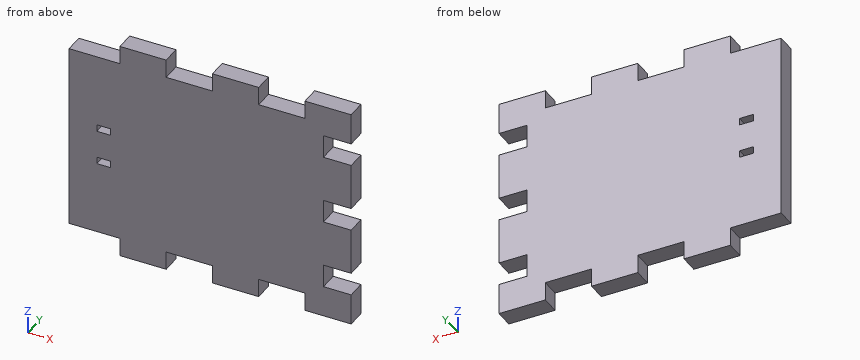
```python
from build123d import *

# Parameters (mm, degrees)
SKETCH1_W           = 55
SKETCH1_H           = 40.5
BOSS_EXTRUDE1_DEPTH = 4
SKETCH2_W           = 2.75
SKETCH2_H           = 4
SKETCH2_W_2         = 10
BOSS_EXTRUDE2_DEPTH = 6
SKETCH3_W           = 10
SKETCH3_H           = 4
BOSS_EXTRUDE3_DEPTH = 4
LPATTERN1_COUNT     = 3
LPATTERN1_PITCH     = 20
SKETCH4_W           = 3
SKETCH4_H           = 1.5
CUT_EXTRUDE1_DEPTH  = 5


with BuildPart() as part:
    # Sketch1 → Boss-Extrude1 (new body)
    with BuildSketch(Plane(origin=(0, 0, 0), x_dir=(1, 0, 0), z_dir=(0, 1, 0))):
        with Locations((27.5, -20.25)):
            Rectangle(SKETCH1_W, SKETCH1_H)
    extrude(amount=BOSS_EXTRUDE1_DEPTH)

    # Sketch2 → Boss-Extrude2 (add)
    with BuildSketch(Plane(origin=(55, 0, 0), x_dir=(0, 0, -1), z_dir=(1, 0, 0))):
        with Locations((-39.125, 2)):
            Rectangle(SKETCH2_W, SKETCH2_H)
        with Locations((-27.75, 2)):
            Rectangle(SKETCH2_W_2, SKETCH2_H)
        with Locations((-12.75, 2)):
            Rectangle(SKETCH2_W_2, SKETCH2_H)
        with Locations((-1.375, 2)):
            Rectangle(SKETCH2_W, SKETCH2_H)
    extrude(amount=BOSS_EXTRUDE2_DEPTH)

    # Sketch3 → Boss-Extrude3 (add, through all)
    with BuildSketch(Plane(origin=(0, 4, 0), x_dir=(1, 0, 0), z_dir=(0, 1, 0))):
        with Locations((56, 2)):
            Rectangle(SKETCH3_W, SKETCH3_H)
        with Locations((56, -42.5)):
            Rectangle(SKETCH3_W, SKETCH3_H)
    boss_extrude3 = extrude(amount=-BOSS_EXTRUDE3_DEPTH)

    # LPattern1: Boss-Extrude3 ×3
    with Locations(*[(-i * LPATTERN1_PITCH, 0, 0) for i in range(1, LPATTERN1_COUNT)]):
        add(boss_extrude3)

    # Sketch4 → Cut-Extrude1 (cut, through all)
    with BuildSketch(Plane(origin=(0, 4, 0), x_dir=(1, 0, 0), z_dir=(0, 1, 0))):
        with Locations((7.5, -24)):
            Rectangle(SKETCH4_W, SKETCH4_H)
        with Locations((7.5, -16.5)):
            Rectangle(SKETCH4_W, SKETCH4_H)
    extrude(amount=-CUT_EXTRUDE1_DEPTH, mode=Mode.SUBTRACT)


solid = part.part
```
Geometry check sheet. Reference: the model listing, model coordinates, mm. Round coordinates to 2 decimals unless told otherwise and drop trailing zeros. Order: outer loops, then holes, each group sorted by start corner. A loop starts at its lowest first (then second) coordinate and runs counter-clockwise, first axis right, second up. Notation, with made-up numbers: (55, 29) - (66, 29) arc R22 ccw to (66, 51) - close; hole circle Ø2 at (0.25, 4). An arc over 180 degrees is marked (long way). Use a Markdown table: item, result. Add a question column.
1) Section check B-B (x = 22.5). Record the cut outline in (y, z), then the cut area to 3 significant figures.
2) Thickness scan on line 1 along X through (y, z) = (3.4, 42.5); line 2 along Z through (x, y) = (7, 0.85); line 3 along X through (y, z) = (2.7, 17). Record the ranges inside material, lowest first.
3) Section check A-A (y = 1.2). Count the separate pieces of the cut face and the enclosed holes in it, then the cut area to 3 significant figures.
4) Section check C-C (z = 35). Record the cut outline in (x, y), then the cut area to 3 significant figures.
5) Gauge pin test, flat ends, axial feed: P1, Ø8, axis at x = 26.5, z = 27, coming from the -Y side; P2, Ø1.2, axis at y = 2, z = 34, coming from the +X side; P3, Ø2, axis at y = 1.5, z = 43.5, coming from the -X side; P4, Ø0.9, axis at x = 7, y = 2.5, coming from the -Z side. Record the tip position at first contact, or that the pin passes through.
Established:
| question | item | result |
|---|---|---|
| 1 | outline | (0, 0) - (4, 0) - (4, 40.5) - (0, 40.5) - close |
| 1 | area | 162 mm2 |
| 2 | line 1 | 11 to 21, 31 to 41, 51 to 61 |
| 2 | line 2 | 0 to 15.75, 17.25 to 23.25, 24.75 to 40.5 |
| 2 | line 3 | 0 to 6, 9 to 61 |
| 3 | separate pieces | 1 |
| 3 | enclosed holes | 2 |
| 3 | area | 2,610 mm2 |
| 4 | outline | (0, 0) - (55, 0) - (55, 4) - (0, 4) - close |
| 4 | area | 220 mm2 |
| 5 | P1 | y = 0 |
| 5 | P2 | x = 55 |
| 5 | P3 | x = 11 |
| 5 | P4 | z = 0 |
